Can you work these out from the model? Positions are in its coordinate system, mm. A direction names the side the tool comes from. Give positions to 0.01 mm unless a question says otherwise; leave off trailing zeros. Write each loop counter-clockwise with the first axis right and the second up, starting at its lowest first coordinate (ties: lowest second). Pieces come first, ordered by that corner, then holes. Notation, with made-up numbers: (20, 77) - (40, 77) arc R32 ccw to (40, 108) - close; hole circle Ø9 at (71.25, -36). An arc over 180 degrees is marked (long way). Use a Markdown table: item, result. Add a question column.
```python
from build123d import *

# Parameters (mm, degrees)
SKETCH_W      = 54
SKETCH_H      = 26
SKETCH_R      = 1.1
SKETCH_W_2    = 9
SKETCH_H_2    = 6.2
PAD_DEPTH     = 2
SKETCH001_W   = 54
SKETCH001_H   = 28
SKETCH001_W_2 = 52
SKETCH001_H_2 = 26
PAD001_DEPTH  = 10
PAD002_DEPTH  = 52
POCKET_DEPTH  = 54.001


with BuildPart() as part:
    # Sketch → Pad (new body)
    with BuildSketch(Plane.XY):
        with Locations((27, 13)):
            Rectangle(SKETCH_W, SKETCH_H)
        with Locations((40.5, 13)):
            Circle(SKETCH_R, mode=Mode.SUBTRACT)
        with Locations((18.5, 13)):
            Rectangle(SKETCH_W_2, SKETCH_H_2, mode=Mode.SUBTRACT)
    extrude(amount=PAD_DEPTH)

    # Sketch001 (on Face11 of Pad) → Pad001 (join)
    with BuildSketch(Plane.XY.offset(2)):
        with Locations((27, 13)):
            Rectangle(SKETCH001_W, SKETCH001_H)
        with Locations((27, 13)):
            Rectangle(SKETCH001_W_2, SKETCH001_H_2, mode=Mode.SUBTRACT)
    extrude(amount=PAD001_DEPTH)

    # Sketch002 (on Face22 of Pad001) → Pad002 (join)
    with BuildSketch(Plane.YZ.offset(1)):
        Polygon((0, 2), (0, 3), (1, 2), align=None)
        Polygon((26, 2), (26, 3), (25, 2), align=None)
    extrude(amount=PAD002_DEPTH)

    # Sketch003 (on Face8 of Pad002) → Pocket (cut, through all)
    with BuildSketch(Plane.YZ.offset(54)):
        Polygon((-1, 2), (-1, 3), (0, 2), align=None)
        Polygon((27, 2), (27, 3), (26, 2), align=None)
    extrude(amount=-POCKET_DEPTH, mode=Mode.SUBTRACT)


solid = part.part
```
Q1. If I drill on probe 1 along X at (y, z) = (23.75, 6); probe 2 along X at (y, z) = (10.5, 1); probe 3 along Y at (x, z) = (40.5, 0.5), over which ranges is the centre line in solid material (lowest first)? Write a range as [from, to].
Q2. If we mould it in two halves opening along X, with no side actions, what happens to faces 1 (the flat face through (14, 13, 1)), 2 (the flat face through (54, 13, 6)), 3 (the flat face through (0, 13, 6)), 4 (the flat face through (27, 0, 1))? For each: released by +X, released by -X, zero draft, split by the parting line, or undercut.
Q3. Suppose I cut it at A-A (y = 13). Please give me the cut outline in (x, z).
Q4. Suppose I cut it at D-D (y = 21). Please give me the cut outline in (x, z).
Q5. I'm going to push flat-ended pins straight in: P1, Ø1.6, axis at x = 17.5, z = 1.5, coming from the +Y side; P2, Ø2, axis at x = 34.5, y = 18.5, coming from the +Z side; P3, Ø0.6, axis at x = 24.5, z = 1, coming from the -Y side. Where does each tip first touch, or does it pass through?
Q6. Suppose I cut it at B-B (z = 8.75). Please give me the cut outline in (x, y).
Q7. Suppose I cut it at C-C (x = 40.5). Please give me the cut outline in (y, z), and give its area (3 significant figures).
Q8. On a 3-axis mill with a long thin cutter (end or side, diameter ignored), from which of +Z, -Z, +X, -X, +Y, -Y can I reach the whole of each face in a straight line? I mean faces 5 (the flat face through (18, 16.1, 1)), 6 (the flat face through (27, 26, 1)), 7 (the flat face through (27, 26, 7)), 8 (the flat face through (27, 13, 0)). Say none if no direction works.
Derived:
| question | item | result |
|---|---|---|
| 1 | probe 1 | [0, 1], [53, 54] |
| 1 | probe 2 | [0, 14], [23, 54] |
| 1 | probe 3 | [0, 11.9], [14.1, 26] |
| 2 | face 1 | undercut |
| 2 | face 2 | released by +X |
| 2 | face 3 | released by -X |
| 2 | face 4 | zero draft |
| 3 | outline | (0, 0) - (14, 0) - (14, 2) - (1, 2) - (1, 12) - (0, 12) - close; (23, 0) - (39.4, 0) - (39.4, 2) - (23, 2) - close; (41.6, 0) - (54, 0) - (54, 12) - (53, 12) - (53, 2) - (41.6, 2) - close |
| 4 | outline | (0, 0) - (54, 0) - (54, 12) - (53, 12) - (53, 2) - (1, 2) - (1, 12) - (0, 12) - close |
| 5 | P1 | y = 26.3 |
| 5 | P2 | z = 2 |
| 5 | P3 | y = 0 |
| 6 | outline | (0, -1) - (54, -1) - (54, 27) - (0, 27) - close; hole (1, 0) - (53, 0) - (53, 26) - (1, 26) - close |
| 7 | outline | (-1, 3) - (0, 2) - (0, 0) - (11.9, 0) - (11.9, 2) - (1, 2) - (0, 3) - (0, 12) - (-1, 12) - close; (14.1, 0) - (26, 0) - (26, 2) - (27, 3) - (27, 12) - (26, 12) - (26, 3) - (25, 2) - (14.1, 2) - close |
| 7 | area | 67.6 mm² |
| 8 | face 5 | +Z, -Z |
| 8 | face 6 | -Z, +X, -X, +Y |
| 8 | face 7 | +Z |
| 8 | face 8 | -Z, +X, -X, +Y, -Y |
